Source: CAD feature listing. Evaluate the final solid. Frame: model axes, mm. A direction names the side the tool comes from. Round coordinates to 2 decimals unless told otherwise and drop trailing zeros. Order: outer loops, then holes, each group sorted by start corner. A loop starts at its lowest first (then second) coordinate and runs counter-clockwise, first axis right, second up. Notation, with made-up numbers: (43, 25.5) -> (97, 25.5) arc R28 ccw to (97, 49.5) -> close; hole circle Ø7 at (37.25, -11). An arc over 180 degrees is marked (long way). One line per item, written item: value. Start each with the question number.
1) Mould query, pull axis Z, two halves, no side actions, for faces 5 (the face through (-20, 28, 15)), 6 (the face through (0, 30, 40)), 7 (the face through (0, 32, 15)). Classes: pulls with the +Z half, pulls with the -Z half, needs draft (parallel to the pull), parting line crosses it, or undercut.
2) Reachability of faces 1 (the face through (-13, 30, 30)), 2 (the face through (-20, 10, 50)), 3 (the face through (19, 10, 50)), 4 (the face through (5, 26, 36)) from +Z, -Z, +X, -X, +Y, -Y: full face, straight path, thin tool, end or side. Return the list, or none.
3) Section B-B (y = 25). Return the cut outline in (x, z), and give its area (3 significant figures).
4) Section C-C (y = 18.5). Return the cut outline in (x, z).
5) Ray query, L1, parallel to X at y = 22.5, z = 5; L2, parallel to X at y = 27.5, z = 38; L3, parallel to Z at x = -6, y = 31. Return the intervals inside material, ascending.
6) Pin query (flat end, axial travel): P1, Ø3.5, axis at x = 19.5, y = 10, coming from the +Z side; P2, Ø22, axis at y = 31.5, z = 12, coming from the -X side; P3, Ø10, axis at y = 28, z = 38.5, coming from the +X side; P4, Ø16, axis at y = 25.5, z = 38, coming from the -X side. Return the tip coordinate at first contact, or that it passes through.
7) Section A-A (x = 0). Return the cut outline in (y, z).
```python
from build123d import *

# Parameters (mm, degrees)
SKETCH1_W           = 50
SKETCH1_H           = 20
BOSS_EXTRUDE1_DEPTH = 50
SKETCH2_W           = 40
SKETCH2_H           = 30
BOSS_EXTRUDE2_DEPTH = 20
CUT_EXTRUDE1_DEPTH  = 79.262379212
BOSS_EXTRUDE3_DEPTH = 20
BOSS_EXTRUDE4_DEPTH = 5


with BuildPart() as part:
    # Sketch1 → Boss-Extrude1 (new body)
    with BuildSketch(Plane.XY):
        with Locations((0, 10)):
            Rectangle(SKETCH1_W, SKETCH1_H)
    extrude(amount=BOSS_EXTRUDE1_DEPTH)

    # Sketch2 → Boss-Extrude2 (add)
    with BuildSketch(Plane(origin=(0, 20, 0), x_dir=(1, 0, 0), z_dir=(0, 1, 0))):
        with Locations((0, -15)):
            Rectangle(SKETCH2_W, SKETCH2_H)
    extrude(amount=BOSS_EXTRUDE2_DEPTH)

    # Sketch3 → Cut-Extrude1 (cut, through all)
    with BuildSketch(Plane(origin=(20, 0, 0), x_dir=(0, 0, -1), z_dir=(1, 0, 0))):
        with BuildLine():
            Line((-23, 40), (-7, 40))
            ThreePointArc((-7, 40), (-15, 32), (-23, 40))
        make_face()
    extrude(amount=-CUT_EXTRUDE1_DEPTH, mode=Mode.SUBTRACT)

    # Sketch4 → Boss-Extrude3 (add)
    with BuildSketch(Plane(origin=(0, 20, 0), x_dir=(1, 0, 0), z_dir=(0, 1, 0))):
        with BuildLine():
            Line((14, -50), (-14, -50))
            ThreePointArc((-14, -50), (0, -64), (14, -50))
        make_face()
    extrude(amount=-BOSS_EXTRUDE3_DEPTH)

    # Sketch5 → Boss-Extrude4 (add, symmetric)
    with BuildSketch(Plane(origin=(0, 0, 0), x_dir=(0, 0, -1), z_dir=(1, 0, 0))):
        Polygon((-30, 20), (-30, 40), (-50, 20), align=None)
    extrude(amount=BOSS_EXTRUDE4_DEPTH, both=True)


solid = part.part
```
Findings:
1. face 5: needs draft
1. face 6: pulls with the +Z half
1. face 7: undercut
2. face 1: +Z, -X, +Y
2. face 2: +Z, -X, +Y, -Y
2. face 3: +Z, +X, +Y, -Y
2. face 4: +Z, +X, +Y
3. outline: (-20, 0) -> (20, 0) -> (20, 30) -> (5, 30) -> (5, 45) -> (-5, 45) -> (-5, 30) -> (-20, 30) -> close
3. area: 1,350 mm2
4. outline: (-25, 0) -> (25, 0) -> (25, 50) -> (14, 50) arc R14 ccw to (-14, 50) -> (-25, 50) -> close
5. L1: -20 to 20
5. L2: -5 to 5
5. L3: 0 to 30
6. P1: z = 50
6. P2: x = -20
6. P3: x = 5
6. P4: x = -25
7. outline: (0, 0) -> (40, 0) -> (40, 7) arc R8 cw to (40, 23) -> (40, 30) -> (20, 50) -> (20, 64) -> (0, 64) -> close
